from build123d import *
from build123d.topology import SkipClean

# Parameters (mm, degrees)
SKETCH1_R           = 14
SKETCH1_R_2         = 2.25
BOSS_EXTRUDE1_DEPTH = 5
SKETCH2_R           = 1.5
CUT_EXTRUDE1_DEPTH  = 21.420577857
SKETCH4_R           = 3.5
CUT_EXTRUDE2_DEPTH  = 3
CIRPATTERN1_COUNT   = 2
SKETCH5_R           = 14
SKETCH5_R_2         = 5
BOSS_EXTRUDE2_DEPTH = 7
SKETCH6_R           = 3.5
CUT_EXTRUDE3_DEPTH  = 22
SKETCH9_OUTSIDE_W   = 38.276
SKETCH9_OUTSIDE_H   = 38.276
SKETCH9_OUTSIDE_W_2 = 24
SKETCH9_OUTSIDE_H_2 = 30
CUT_EXTRUDE5_DEPTH  = 7
SKETCH10_R          = 1.5
CUT_EXTRUDE6_DEPTH  = 32.874754901
SKETCH12_W          = 4.5
SKETCH12_H          = 18
CUT_EXTRUDE7_DEPTH  = 7
CHAMFER2_SIZE       = 0.4
CHAMFER2_SIZE2      = 4.572020921
FILLET2_R           = 1
CHAMFER3_SIZE       = 1


# Some blends are built 0.0001 mm under size
with BuildPart() as part:
    # Sketch1 → Boss-Extrude1 (new body)
    with BuildSketch(Plane(origin=(0, 0, 0), x_dir=(1, 0, 0), z_dir=(0, 1, 0))):
        with Locations(Location((0, 0, 0), (0, 0, 270))):
            Circle(SKETCH1_R)
        with Locations(Location((0, 0, 0), (0, 0, 270))):
            Circle(SKETCH1_R_2, mode=Mode.SUBTRACT)
    extrude(amount=BOSS_EXTRUDE1_DEPTH)

    # Sketch2 → Cut-Extrude1 (cut, through all)
    with BuildSketch(Plane(origin=(0, 5, 0), x_dir=(1, 0, 0), z_dir=(0, 1, 0))):
        with Locations(Location((0, 9, 0), (0, 0, 270))):
            Circle(SKETCH2_R)
    cut_extrude1 = extrude(amount=-CUT_EXTRUDE1_DEPTH, mode=Mode.SUBTRACT)

    # Sketch4 → Cut-Extrude2 (cut)
    with BuildSketch(Plane(origin=(0, 5, 0), x_dir=(1, 0, 0), z_dir=(0, 1, 0))):
        with Locations(Location((0, 9, 0), (0, 0, 270))):
            Circle(SKETCH4_R)
    cut_extrude2 = extrude(amount=-CUT_EXTRUDE2_DEPTH, mode=Mode.SUBTRACT)

    # CirPattern1: Cut-Extrude1, Cut-Extrude2 ×2 about axis
    cirpattern1_axis = Axis((0, 0, 0), (0, 1, 0))
    add([cut_extrude1.rotate(cirpattern1_axis, i * 360 / CIRPATTERN1_COUNT) for i in range(1, CIRPATTERN1_COUNT)], mode=Mode.SUBTRACT)
    add([cut_extrude2.rotate(cirpattern1_axis, i * 360 / CIRPATTERN1_COUNT) for i in range(1, CIRPATTERN1_COUNT)], mode=Mode.SUBTRACT)

    # Sketch5 → Boss-Extrude2 (add)
    with BuildSketch(Plane(origin=(0, 5, 0), x_dir=(1, 0, 0), z_dir=(0, 1, 0))):
        with Locations(Location((0, 0, 0), (0, 0, 270))):
            Circle(SKETCH5_R)
        with Locations(Location((0, 0, 0), (0, 0, 270))):
            Circle(SKETCH5_R_2, mode=Mode.SUBTRACT)
    extrude(amount=BOSS_EXTRUDE2_DEPTH)

    # Sketch6 → Cut-Extrude3 (cut, through all)
    with SkipClean():  # the faces are left unmerged after this step: merging them gives an invalid solid
        with BuildSketch(Plane(origin=(0, 5, 0), x_dir=(1, 0, 0), z_dir=(0, 1, 0))):
            with Locations(Location((0, 9, 0), (0, 0, 270))):
                Circle(SKETCH6_R)
            with Locations(Location((0, -9, 0), (0, 0, 270))):
                Circle(SKETCH6_R)
        extrude(amount=CUT_EXTRUDE3_DEPTH, mode=Mode.SUBTRACT)

    # Sketch9 outside → Cut-Extrude5 (cut)
    with SkipClean():  # the faces are left unmerged after this step: merging them gives an invalid solid
        with BuildSketch(Plane(origin=(0, 12, 0), x_dir=(1, 0, 0), z_dir=(0, 1, 0))):
            Rectangle(SKETCH9_OUTSIDE_W, SKETCH9_OUTSIDE_H)
            Rectangle(SKETCH9_OUTSIDE_W_2, SKETCH9_OUTSIDE_H_2, mode=Mode.SUBTRACT)
        extrude(amount=-CUT_EXTRUDE5_DEPTH, mode=Mode.SUBTRACT)

    # Sketch10 → Cut-Extrude6 (cut, through all)
    with SkipClean():  # the faces are left unmerged after this step: merging them gives an invalid solid
        with BuildSketch(Plane(origin=(12, 0, 0), x_dir=(0, 0, -1), z_dir=(1, 0, 0))):
            with Locations((0, 8.75)):
                Circle(SKETCH10_R)
        extrude(amount=-CUT_EXTRUDE6_DEPTH, mode=Mode.SUBTRACT)

    # Sketch12 → Cut-Extrude7 (cut)
    with SkipClean():  # the faces are left unmerged after this step: merging them gives an invalid solid
        with BuildSketch(Plane(origin=(0, 12, 0), x_dir=(1, 0, 0), z_dir=(0, 1, 0))):
            Rectangle(SKETCH12_W, SKETCH12_H)
        extrude(amount=-CUT_EXTRUDE7_DEPTH, mode=Mode.SUBTRACT)
    add(part.part.scale(1), mode=Mode.REPLACE)  # the faces are merged on a copy

    # Chamfer2
    chamfer2_edges = [part.edges().sort_by_distance(p)[0] for p in [
        (1.59099026, 5, 1.590990255),
    ]]
    chamfer2_side = [part.faces().sort_by_distance(p)[0] for p in [
        (0, 5, 3.259288519),
    ]]
    chamfer(chamfer2_edges, length=CHAMFER2_SIZE, length2=CHAMFER2_SIZE2, reference=chamfer2_side[0])

    # Fillet2
    # the kernel refuses this fillet: 1 mm, written as the material it takes off along each edge
    with BuildSketch(Plane(origin=(2.25, 13.446043689, -4.465142775), x_dir=(0, 0, -1), z_dir=(0, -1, 0)), Plane(origin=(-2.25, 13.446043689, 4.465142775), x_dir=(0, 0, 1), z_dir=(0, -1, 0))) as fillet2_piece_1:
        with BuildLine():
            CenterArc((0.578417476, 1), FILLET2_R, 212.797168296, 57.202831704)
            ThreePointArc((-0.262175899, 0.458333333), (-0.125033492, 0.232629939), (0, 0))
            Line((0, 0), (0.578417476, 0))
        make_face()
    extrude(amount=8.446043689, mode=Mode.SUBTRACT)
    with BuildSketch(Plane(origin=(2.25, 13.446043689, 4.465142775), x_dir=(0.8680218565985627, 0, -0.49652598770576395), z_dir=(0, -1, 0))) as fillet2_piece_2:
        with BuildLine():
            CenterArc((0.580822548, 0.998604999), FILLET2_R, 209.770426123, 57.202831704)
            Line((-0.287199308, 0.502079011), (0, 0))
            ThreePointArc((0, 0), (0.264010249, 0.006975006), (0.528020498, 0))
        make_face()
    extrude(amount=8.446043689, mode=Mode.SUBTRACT)
    with BuildSketch(Plane(origin=(-2.25, 13.446043689, -4.465142775), x_dir=(0, 0, -1), z_dir=(0, -1, 0))) as fillet2_piece_3:
        with BuildLine():
            CenterArc((0.578417476, -1), FILLET2_R, 90, 57.202831704)
            ThreePointArc((-0.262175899, -0.458333333), (-0.125033492, -0.232629939), (0, 0))
            Line((0, 0), (0.578417476, 0))
        make_face()
    extrude(amount=8.446043689, mode=Mode.SUBTRACT)
    with BuildSketch(Plane(origin=(-2.25, 13.07880894, -6.319048676), x_dir=(0, 0, 1), z_dir=(0, -1, 0))) as fillet2_piece_4:
        with BuildLine():
            CenterArc((0.431523576, 1), FILLET2_R, 226.238257307, 43.761742693)
            ThreePointArc((-0.260137513, 0.277777778), (-0.126290486, 0.14242722), (0, 0))
            Line((0, 0), (0.431523576, 0))
        make_face()
    extrude(amount=8.07880894, mode=Mode.SUBTRACT)
    with BuildSketch(Plane(origin=(-2.25, 13.07880894, 6.319048676), x_dir=(-0.7299030964550425, 0, 0.683550634397585), z_dir=(0, -1, 0)), Plane(origin=(2.25, 13.07880894, -6.319048676), x_dir=(0.7299030964550413, 0, -0.6835506343975865), z_dir=(0, -1, 0))) as fillet2_piece_5:
        with BuildLine():
            CenterArc((0.434934882, 0.998521029), FILLET2_R, 223.121729096, 43.761742693)
            Line((-0.294968214, 0.314970394), (0, 0))
            ThreePointArc((0, 0), (0.190284011, 0.0051764), (0.380568022, 0))
        make_face()
    extrude(amount=8.07880894, mode=Mode.SUBTRACT)
    with BuildSketch(Plane(origin=(2.25, 13.07880894, 6.319048676), x_dir=(0.7299030964550418, 0, 0.6835506343975857), z_dir=(0, -1, 0))) as fillet2_piece_6:
        with BuildLine():
            CenterArc((0.434934882, -0.998521029), FILLET2_R, 93.116528211, 43.761742693)
            Line((-0.294968214, -0.314970394), (0, 0))
            ThreePointArc((0, 0), (0.190284011, -0.0051764), (0.380568022, 0))
        make_face()
    extrude(amount=8.07880894, mode=Mode.SUBTRACT)

    # Chamfer3
    chamfer3_edges = [part.edges().sort_by_distance(p)[0] for p in [
        (-2.372028854, 12, -4.564846697),
        (5, 12, 0),
        (2.372028854, 12, -4.564846697),
        (2.25, 12, -5.465542675),
        (2.322039273, 12, -6.260203097),
        (0, 12, -12.5),
        (-2.322039273, 12, -6.260203097),
        (-2.25, 12, -5.465542675),
        (-5, 12, 0),
        (-2.372028854, 12, 4.564846697),
        (-2.25, 12, 5.465542675),
        (-2.322039273, 12, 6.260203097),
        (-3.218916614, 12, 10.374254646),
        (3.218916614, 12, 10.374254646),
        (2.322039273, 12, 6.260203097),
        (2.25, 12, 5.465542675),
        (2.372028854, 12, 4.564846697),
    ]]
    chamfer(chamfer3_edges, length=CHAMFER3_SIZE - 0.0001)  # a hair under: the kernel refuses the full size
    chamfer3_2_edges = [part.edges().sort_by_distance(p)[0] for p in [
        (-14, 5, 0),
    ]]
    chamfer(chamfer3_2_edges, length=CHAMFER3_SIZE)
    chamfer3_3_edges = [part.edges().sort_by_distance(p)[0] for p in [
        (14, 5, 0),
    ]]
    chamfer(chamfer3_3_edges, length=CHAMFER3_SIZE)
    chamfer3_4_edges = [part.edges().sort_by_distance(p)[0] for p in [
        (-12, 12, 0),
    ]]
    chamfer(chamfer3_4_edges, length=CHAMFER3_SIZE)
    chamfer3_5_edges = [part.edges().sort_by_distance(p)[0] for p in [
        (12, 12, 0),
    ]]
    chamfer(chamfer3_5_edges, length=CHAMFER3_SIZE)
    # the kernel refuses this chamfer: 1 mm, written as the material it takes off along each edge
    with BuildSketch(Plane(origin=(0, 12, 0), x_dir=(-0.8854986236945603, 0, 0.46464199921556715), z_dir=(-0.46464199921556715, 0, -0.8854986236945603))) as chamfer3_6_piece_1:
        with BuildLine():
            Line((14.028284271, -1.028284271), (12.971715729, 0.028284271))
            Line((12.971715729, 0.028284271), (12.971715729, 0.048284271))
            ThreePointArc((12.971715729, 0.048284271), (13.485857864, 0.02), (14, 0.02))
            Line((14, 0.02), (14.02, 0))
            ThreePointArc((14.02, 0), (14.02, -0.514142136), (14.048284271, -1.028284271))
            Line((14.048284271, -1.028284271), (14.028284271, -1.028284271))
        make_face()
    revolve(axis=Axis((0, 12, 0), (0, 1, 0)), revolution_arc=62.312944684, mode=Mode.SUBTRACT)
    with BuildSketch(Plane(origin=(0, 12, 0), x_dir=(0, 0, 1), z_dir=(-1, 0, 0))) as chamfer3_6_piece_2:
        with BuildLine():
            Line((14.028284271, -1.028284271), (12.971715729, 0.028284271))
            Line((12.971715729, 0.028284271), (12.971715729, 0.048284271))
            ThreePointArc((12.971715729, 0.048284271), (13.485857864, 0.02), (14, 0.02))
            Line((14, 0.02), (14.02, 0))
            ThreePointArc((14.02, 0), (14.02, -0.514142136), (14.048284271, -1.028284271))
            Line((14.048284271, -1.028284271), (14.028284271, -1.028284271))
        make_face()
    revolve(axis=Axis((0, 12, 0), (0, 1, 0)), revolution_arc=62.312944684, mode=Mode.SUBTRACT)
    # the kernel refuses this chamfer: 1 mm, written as the material it takes off along each edge
    with BuildSketch(Plane(origin=(0, 12, 0), x_dir=(0.8855326835196512, 0, -0.46457708339788484), z_dir=(0.46457708339788484, 0, 0.8855326835196512))) as chamfer3_7_piece_1:
        with BuildLine():
            Line((14.028284271, -1.028284271), (12.971715729, 0.028284271))
            Line((12.971715729, 0.028284271), (12.971715729, 0.048284271))
            ThreePointArc((12.971715729, 0.048284271), (13.485857864, 0.02), (14, 0.02))
            Line((14, 0.02), (14.02, 0))
            ThreePointArc((14.02, 0), (14.02, -0.514142136), (14.048284271, -1.028284271))
            Line((14.048284271, -1.028284271), (14.028284271, -1.028284271))
        make_face()
    revolve(axis=Axis((0, 12, 0), (0, 1, 0)), revolution_arc=124.634289903, mode=Mode.SUBTRACT)


solid = part.part
Design review of the part built by this model. Coordinates are the model's own, in mm. A direction names the side the tool comes from. Coordinates: 2 decimals unless noted, no trailing zeros. Write each loop counter-clockwise with the first axis right and the second up, starting at its lowest first coordinate (ties: lowest second). Pieces come first, ordered by that corner, then holes. Notation, with made-up numbers: (-40, 63.25) -> (-16, 63.25) arc R11 ccw to (-16, 72.25) -> close; hole circle Ø8 at (-21, 1). An arc over 180 degrees is marked (long way). Write each question's results on one line, items separated by ' | '. Start each with the question number.
(1) For line 1 along Y through (x, z) = (-7, 0); line 2 along Z through (x, y) = (5, 8.75); line 3 along X through (y, z) = (3.75, -9), list the stretches that pass through material, from the lowest coordinate up. Write a range as from..to.
(2) Take a section at B-B on y = 8.75. Write out the cut boundary in (x, z), and give its area (3 significant figures).
(3) Take a section at A-A on y = 5.5. Write out the cut boundary in (x, z).
(4) Clearance check with flat-ended pins moving along their axes: P1, Ø0.7, axis at y = 8, z = -5.5, coming from the +X side; P2, Ø3.5, axis at y = 8.75, z = 0, coming from the -X side; P3, Ø4, axis at y = 4.5, z = 11, coming from the -X side. State where each tip first meets the part, or that it passes through.
(5) The part is to be moulded in two halves that separate along Z. For faces 3 (the face through (-13.3, 4.7, 0.1)), 4 (the face through (-8, 12, 0)), 5 (the face through (0.035, 2.682, -2.447)), 6 (the face through (2.76, 11.51, 5.46)), say which applies: pulls with the +Z half, pulls with the -Z half, needs draft (parallel to the pull), parting line crosses it, or undercut.
(6) Take a section at C-C on z = 0. Give the number of separate pieces and of enclosed holes in the cut face, and give its area (3 significant figures).
(7) Tool access review of faces 1 (the face through (-0.07, 1.01, 10.5)), 2 (the face through (0.154, 6.563, -12.497)): name each direction out of +Z, -Z, +X, -X, +Y, -Y from which nothing blocks a thin tool from reaching the whole face with its end or side.
Results found:
1) line 1: y = 0..7.25, 10.25..12 | line 2: z = -13.08..-1.5, 1.5..13.08 | line 3: x = -10.72..-3.5, 3.5..10.72
2) outline: (-12, -7.21) arc R14 ccw to (12, -7.21) -> (12, -1.5) -> (4.77, -1.5) arc R5 cw to (2.71, -4.2) arc R1 ccw to (2.25, -5.04) -> (2.25, -5.89) arc R1 ccw to (2.53, -6.58) arc R3.5 cw (long way) to (-2.53, -6.58) arc R1 ccw to (-2.25, -5.89) -> (-2.25, -5.04) arc R1 ccw to (-2.71, -4.2) arc R5 cw to (-4.77, -1.5) -> (-12, -1.5) -> close; (-12, 1.5) -> (-4.77, 1.5) arc R5 cw to (-2.71, 4.2) arc R1 ccw to (-2.25, 5.04) -> (-2.25, 5.89) arc R1 ccw to (-2.53, 6.58) arc R3.5 cw (long way) to (2.53, 6.58) arc R1 ccw to (2.25, 5.89) -> (2.25, 5.04) arc R1 ccw to (2.71, 4.2) arc R5 cw to (4.77, 1.5) -> (12, 1.5) -> (12, 7.21) arc R14 ccw to (-12, 7.21) -> close | area: 370 mm2
3) outline: (-12, -7.21) arc R14 ccw to (12, -7.21) -> (12, 7.21) arc R14 ccw to (-12, 7.21) -> close; hole (-2.71, -4.2) arc R1 cw to (-2.25, -5.04) -> (-2.25, -5.89) arc R1 cw to (-2.53, -6.58) arc R3.5 ccw (long way) to (2.53, -6.58) arc R1 cw to (2.25, -5.89) -> (2.25, -5.04) arc R1 cw to (2.71, -4.2) arc R5 ccw to (2.71, 4.2) arc R1 cw to (2.25, 5.04) -> (2.25, 5.89) arc R1 cw to (2.53, 6.58) arc R3.5 ccw (long way) to (-2.53, 6.58) arc R1 cw to (-2.25, 5.89) -> (-2.25, 5.04) arc R1 cw to (-2.71, 4.2) arc R5 ccw to start
4) P1: stops at x = 12 | P2: stops at x = -12 | P3: stops at x = -10.72
5) face 3: parting line crosses it | face 4: needs draft | face 5: undercut | face 6: undercut
6) separate pieces: 4 | enclosed holes: 0 | area: 169 mm2
7) face 1: +Y, -Y | face 2: +Y
